For this review, use the dimensioned drawing (mm, ordinates from the lowest corner) and the shaded views. A direction names the side the tool comes from. Coordinates: 2 decimals unless noted, no trailing zeros. Write each loop counter-clockwise with the first axis right and the second up, starting at its lowest first coordinate (ties: lowest second). Pieces come first, ordered by that corner, then holes.
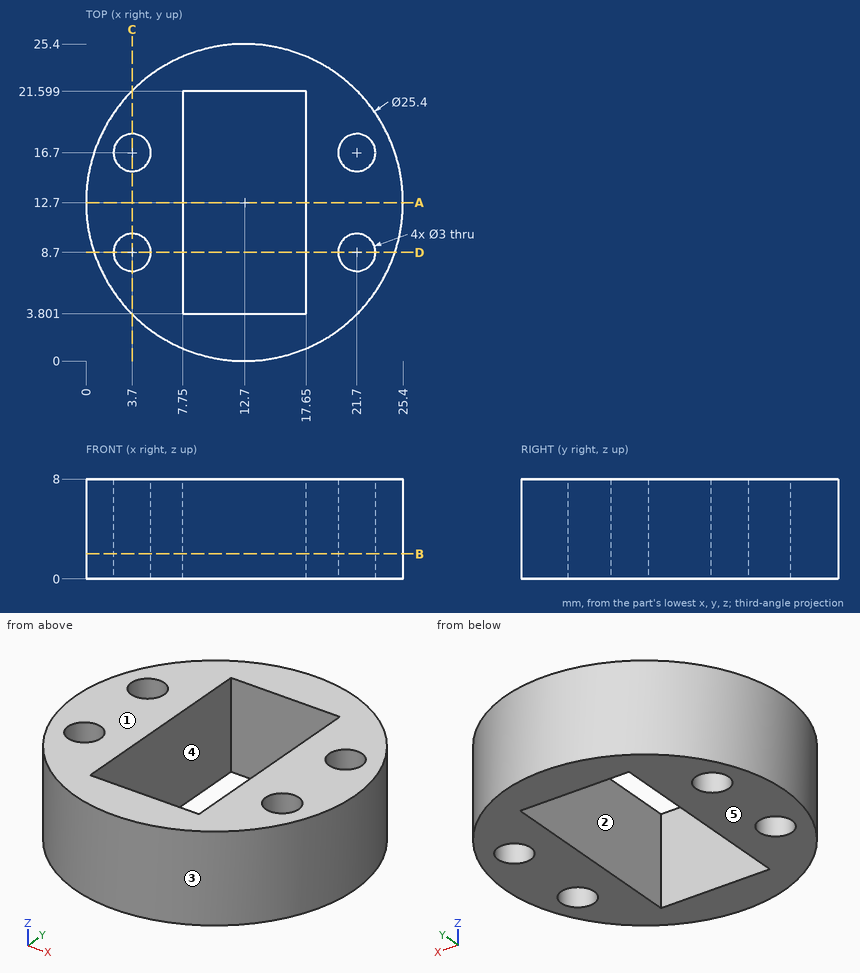
(1) For the marked faces 1 and 2, list the 3-axis set-ups (+Z, -Z, +X, -X, +Y, -Y) from which the entire face can be reached by the end or side of a thin tool; tool diameter is ignored.
(2) Mouldability with a two-part tool opening along Y and no side actions: class the marked faces 3, 4 and 5 as +Y half, -Y half, draft (parallel to the pull), parting line (faces both ways), or undercut.
(3) Consider section A-A (y = 12.7). Give the boundary of the cut face in (x, z).
(4) Consider section D-D (y = 8.7). Give the boundary of the cut face in (x, z).
(5) Insertion check: pin 1 Ø1.5 at (y, z) = (18.5, 1) entering from -X; pin 2 Ø2 at (y, z) = (4.5, 2) entering from -X; pin 3 Ø1.5 at (y, z) = (3, 5.5) entering from +X. Each pin has a flat end and moves straight along its axis. Give the tip position at first contact, or say it passes through.
(6) Consider section C-C (x = 3.7). Give the boundary of the cut face in (y, z).
(7) Consider section B-B (z = 2). Give the boundary of the cut face in (x, y).
(8) Wall thickness on line 1 (Y direction, x = 3.7, z = 4.25); line 2 (Y direction, x = 2.5, z = 5.75) (1 decimal); line 3 (X direction, y = 19.25, z = 2.5): over which ranges is each line inside the solid? List them lowest first.
Results:
1. face 1: +Z, +X, -X, +Y, -Y
1. face 2: +Z, -Z
2. face 3: parting line
2. face 4: undercut
2. face 5: draft
3. outline: (0, 0) - (7.75, 0) - (7.75, 8) - (0, 8) - close; (17.65, 0) - (25.4, 0) - (25.4, 8) - (17.65, 8) - close
4. outline: (0.65, 0) - (2.2, 0) - (2.2, 8) - (0.65, 8) - close; (5.2, 0) - (7.75, 0) - (7.75, 8) - (5.2, 8) - close; (17.65, 0) - (20.2, 0) - (20.2, 8) - (17.65, 8) - close; (23.2, 0) - (24.75, 0) - (24.75, 8) - (23.2, 8) - close
5. pin 1: stops at x = 1.05
5. pin 2: stops at x = 2.24
5. pin 3: stops at x = 21.71
6. outline: (3.74, 0) - (7.2, 0) - (7.2, 8) - (3.74, 8) - close; (10.2, 0) - (15.2, 0) - (15.2, 8) - (10.2, 8) - close; (18.2, 0) - (21.66, 0) - (21.66, 8) - (18.2, 8) - close
7. outline: circle Ø25.4 at (12.7, 12.7); hole circle Ø3 at (3.7, 8.7); hole circle Ø3 at (3.7, 16.7); hole (7.75, 3.8) - (17.65, 3.8) - (17.65, 21.6) - (7.75, 21.6) - close; hole circle Ø3 at (21.7, 8.7); hole circle Ø3 at (21.7, 16.7)
8. line 1: y = 3.74 to 7.2, 10.2 to 15.2, 18.2 to 21.66
8. line 2: y = 5.1 to 7.8, 9.6 to 15.8, 17.6 to 20.3
8. line 3: x = 1.82 to 7.75, 17.65 to 23.58
